Verification items for the finished model (mm, model axes). Face numbers are marked on the shaded views. A direction names the side the tool comes from. Give positions to 0.01 mm unless a question says otherwise; leave off trailing zeros. Loops run counter-clockwise (first coordinate to the right, second up) from the corner with the lowest first, then second, coordinate; pieces in that order, holes last. Notation, with made-up numbers: (12, 49.5) - (46, 49.5) arc R20 ccw to (46, 65.5) - close; hole circle Ø10 at (-33, 33.5). An arc over 180 degrees is marked (long way). Answer in a Markdown table with one row per item.
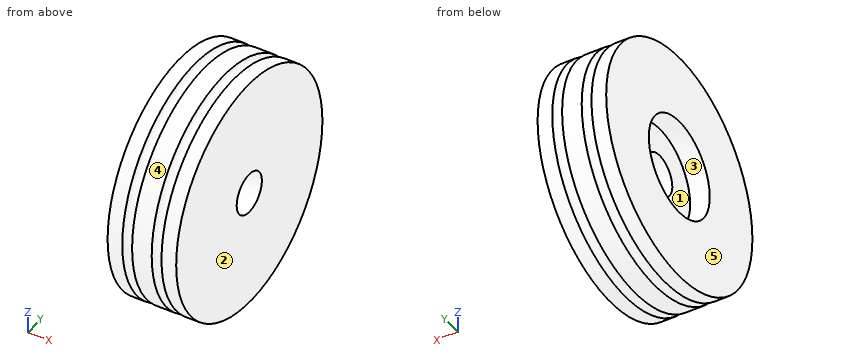
Autodesk Inventor part; units mm, degrees
ref_plane "YZ Plane" through (0, 0, 0) normal (1, 0, 0) x (0, 1, 0)
ref_plane "XZ Plane" through (0, 0, 0) normal (0, 1, 0) x (-1, 0, 0)
ref_plane "XY Plane" through (0, 0, 0) normal (0, 0, 1) x (1, 0, 0)
sketch "Sketch1" plane through (0, 0, 0) normal (0, 0, 1) x (1, 0, 0)
  line L0 (0, 0) -> (0, 12)
  line L1 (0, 12) -> (1.5, 12)
  line L2 (1.5, 12) -> (1.5, 12)
  line L3 (2.5, 12) -> (2.5, 12)
  line L4 (2.5, 12) -> (4.5, 12)
  line L5 (4.5, 12) -> (4.5, 12)
  line L6 (5.5, 12) -> (5.5, 12)
  line L7 (5.5, 12) -> (7, 12)
  line L8 (7, 12) -> (7, 0)
  line L9 (7, 0) -> (0, 0)
  arc A0 (1.5, 12) -> (2.5, 12) centre (2, 12) ccw
  arc A1 (4.5, 12) -> (5.5, 12) centre (5, 12) ccw
  point P0 (0.75, 12)
  dimension "d0" = 7
  dimension "d2" = 0.5
  dimension "d3" = 0.5
  dimension "d4" = 2
  dimension "d5" = 2
  dimension "d6" = 24
revolve "Revolution1" add sketch "Sketch1" angle 360 about axis through (7, 0, 0) along (-1, 0, 0)
sketch "Sketch2" plane through (0, 0, 0) normal (-1, 0, 0) x (0, 0, 1)
  circle A0 centre (0, 0) radius 12
  point P0 (0, 0)
hole "Hole1" at (0, 0, 0) direction (1, 0, 0) diameter 10 depth 2
sketch "Sketch3" plane through (7, 0, 0) normal (1, 0, 0) x (0, 0, -1)
  circle A0 centre (0, 0) radius 12
hole "Hole2" at (7, 0, 0) direction (-1, 0, 0) diameter 4.134 depth 5
equation "\"d5\" = d4"
properties part number "40"
Q1. Sectioned sample at C-C (x = 0.5). Record the cut outline in (y, z).
Completed:
| item | result |
|---|---|
| outline | circle Ø24 at (0, 0); hole circle Ø10 at (0, 0) |
Q2. Tool access check on the marked faces 1 and 2. Record the directions out of +Z, -Z, +X, -X, +Y, -Y that give a thin tool (end or side, any length) a straight path to the whole face; none if there is none.
Completed:
| item | result |
|---|---|
| face 1 | -X |
| face 2 | +Z, -Z, +X, +Y, -Y |
Q3. Go/stop test with flat-tipped pins: P1, Ø3, axis at x = 5.5, z = -3, coming from the +Y side; P2, Ø1, axis at x = 4, y = -8.5, coming from the -Z side; P3, Ø4, axis at x = 3, y = -2.5, coming from the -Z side. Record where each tip stops, or that it passes through.
Completed:
| item | result |
|---|---|
| P1 | y = 11.91 |
| P2 | z = -8.94 |
| P3 | z = -11.99 |
Q4. Thickness scan on line 1 (Y direction, x = 1, z = 0); line 2 (Y direction, x = 4.3, z = 0). Record the ranges inside material, lowest first.
Completed:
| item | result |
|---|---|
| line 1 | -12 to -5, 5 to 12 |
| line 2 | -12 to -2.07, 2.07 to 12 |
Q5. Draft check along Z on the marked faces 3, 4 and 5. Enter one of: +Z half, -Z half, draft (parallel to the pull), parting line (faces both ways), or undercut.
Completed:
| item | result |
|---|---|
| face 3 | undercut |
| face 4 | parting line |
| face 5 | draft |
Q6. Sectioned sample at A-A (y = 0). Record the cut outline in (x, z).
Completed:
| item | result |
|---|---|
| outline | (0, -12) - (1.5, -12) arc R0.5 cw to (2.5, -12) - (4.5, -12) arc R0.5 cw to (5.5, -12) - (7, -12) - (7, -2.07) - (2, -2.07) - (2, -5) - (0, -5) - close; (0, 5) - (2, 5) - (2, 2.07) - (7, 2.07) - (7, 12) - (5.5, 12) arc R0.5 cw to (4.5, 12) - (2.5, 12) arc R0.5 cw to (1.5, 12) - (0, 12) - close |
Q7. Sectioned sample at D-D (x = 3). Record the cut outline in (y, z).
Completed:
| item | result |
|---|---|
| outline | circle Ø24 at (0, 0); hole circle Ø4.13 at (0, 0) |
